Autodesk Inventor part; units mm, degrees
ref_plane "YZ Plane" through (0, 0, 0) normal (1, 0, 0) x (0, 1, 0)
ref_plane "XZ Plane" through (0, 0, 0) normal (0, 1, 0) x (-1, 0, 0)
ref_plane "XY Plane" through (0, 0, 0) normal (0, 0, 1) x (1, 0, 0)
sketch "スケッチ1" plane through (0, 0, 0) normal (0, 1, 0) x (-1, 0, 0)
  line L0 (0, 0) -> (-230, 0)
  line L1 (-230, 0) -> (-230, -35)
  line L2 (-230, -35) -> (0, -35)
  line L3 (0, -35) -> (0, 0)
  arc A0 (0, -35) -> (0, 0) centre (0, -17.5) ccw
  dimension "d0" = 230
  dimension "d1" = 35
  dimension "d2" = 17.5
extrude "押し出し1" add sketch "スケッチ1" along normal blind 3
sketch "スケッチ2" plane through (0, 3, 0) normal (0, 1, 0) x (1, 0, 0)
  line L0 (0, 17.5) -> (238.6526, 17.5)
  line L1 (0, 0) -> (230, 0)
  arc A0 (0, 35) -> (0, 0) centre (0, 17.5) ccw
  point P0 (90, 17.5)
  point P1 (100, 17.5)
  point P2 (110, 17.5)
  point P3 (120, 17.5)
  point P4 (130, 17.5)
  point P5 (140, 17.5)
  point P6 (150, 17.5)
  point P7 (160, 17.5)
  point P8 (170, 17.5)
  point P9 (180, 17.5)
  point P10 (190, 17.5)
  point P11 (200, 17.5)
  point P12 (210, 17.5)
  point P13 (-17.5, 17.5)
  point P14 (220, 17.5)
  point P15 (80, 17.5)
  dimension "d5" = 17.5
  dimension "d13" = 10
  dimension "d14" = 10
  dimension "d15" = 10
  dimension "d16" = 10
  dimension "d17" = 10
  dimension "d18" = 10
  dimension "d19" = 10
  dimension "d20" = 10
  dimension "d21" = 10
  dimension "d22" = 10
  dimension "d23" = 10
  dimension "d24" = 10
  dimension "d35" = 17.5
  dimension "d67" = 10
  dimension "d78" = 10
  dimension "d96" = 80
hole "穴1" at (90, 3, -17.5) at (100, 3, -17.5) at (110, 3, -17.5) at (120, 3, -17.5) at (130, 3, -17.5) at (140, 3, -17.5) at (150, 3, -17.5) at (160, 3, -17.5) at (170, 3, -17.5) at (180, 3, -17.5) at (190, 3, -17.5) at (200, 3, -17.5) at (210, 3, -17.5) at (220, 3, -17.5) at (80, 3, -17.5) direction (0, -1, 0) diameter 3.2 end through all
sketch "スケッチ3" plane through (0, 3, 0) normal (0, 1, 0) x (1, 0, 0)
  line L0 (230, 35) -> (0, 35)
  point P0 (0, 0)
  point P1 (0, 17.5)
  dimension "d36" = 17.5
hole "穴2" at (0, 3, -17.5) direction (0, -1, 0) diameter 16 end through all
sketch "スケッチ4" plane through (0, 3, 0) normal (0, 1, 0) x (1, 0, 0)
  circle A0 centre (0, 17.5) radius 6
  circle A1 centre (0, 17.5) radius 8
  line L0 (-0.1439, 17.5) -> (-6.5454, 17.5)
  line L1 (-6.5454, 17.5) -> (7.5104, 17.5)
  point P0 (0, 0)
  point P1 (0, 11.5)
  point P2 (6, 17.5)
  point P3 (0, 23.5)
  point P4 (-6, 17.5)
  dimension "d44" = 12
  dimension "d45" = 0
hole "穴3" [suppressed]
sketch "スケッチ5" plane through (0, 3, 0) normal (0, 1, 0) x (1, 0, 0)
  circle A0 centre (0, 17.5) radius 8
  point P0 (0, 0)
  point P1 (15.8, 7)
  point P2 (15.8, 28)
  point P3 (24.9999, 17.5)
  dimension "d53" = 10.5
  dimension "d55" = 15.8
  dimension "d56" = 15.8
  dimension "d83" = 10.5
hole "穴4" at (15.8, 3, -28) at (15.8, 3, -7) direction (0, -1, 0) diameter 3.2 end through all
sketch "スケッチ6" plane through (0, 3, 0) normal (0, 1, 0) x (1, 0, 0)
  circle A0 centre (0, 17.5) radius 8 construction
  line L0 (0, 17.5) -> (230, 17.5) construction
  line L1 (230, 0) -> (230, 35) construction
  point P0 (0, 0)
  point P1 (67, 17.5)
  point P2 (47, 17.5)
  dimension "d69" = 47
  dimension "d70" = 20
hole "穴5" at (67, 3, -17.5) at (47, 3, -17.5) direction (0, -1, 0) diameter 6.4 end through all
sketch "スケッチ7" plane through (0, 3, 0) normal (0, 1, 0) x (1, 0, 0)
  circle A0 centre (0, 17.5) radius 8 construction
  circle A1 centre (0, 17.5) radius 12.5 construction
  point P0 (0, 0)
  point P1 (0, 5)
  point P2 (12.5, 17.5)
  point P3 (0, 30)
  point P4 (-12.5, 17.5)
  dimension "d84" = 25
  dimension "d87" = 360
hole "穴6" [suppressed]
properties part number "shoulder2_lower_left_plate" material "アルミニウム 5052"
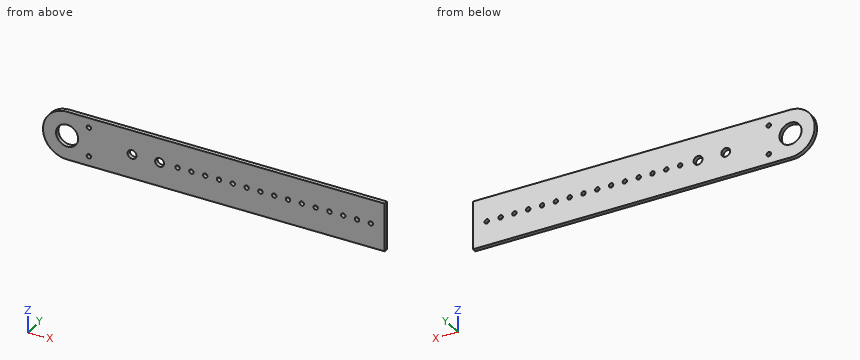
CAD build for the part. Positions are in the model's coordinates, mm. Coordinates: 2 decimals unless noted, no trailing zeros. Write each loop counter-clockwise with the first axis right and the second up, starting at its lowest first coordinate (ties: lowest second). Pieces come first, ordered by that corner, then holes. Notation, with made-up numbers: (85.25, 68) - (135.25, 68) arc R12 cw to (135.25, 80) - close; hole circle Ø1 at (62.5, 27). An arc over 180 degrees is marked (long way). Use a Markdown table: item, result. Add a question column.
Item 1: Band-saw the part on B-B, the plane y = 1.75. Give the number of separate pieces and of enclosed holes in the cut face, and give its area (3 significant figures).
Item 2: Flat gauge pin, fed straight in: pin 1 (1.9 mm diameter, centred on x = 90, z = -17.5, fed in from +Y). Where does the tip first touch, or does it go through?
Item 3: Band-saw the part on A-A, the plane x = 47. Give the cut face in (y, z).
Item 4: Drill centre lines: L1, parallel to Z at x = 47, y = 1.1; L2, parallel to Z at x = 150, y = 0.6; L3, parallel to X at y = 1.6, z = -15.5. Where is each one in solid material? Low to high. Write a range as from..to.
Item 5: Band-saw the part on C-C, the plane z = -3. Give the cut face in (x, y).
Numbers:
| question | item | result |
|---|---|---|
| 1 | separate pieces | 1 |
| 1 | enclosed holes | 20 |
| 1 | area | 8,130 mm2 |
| 2 | pin 1 | through |
| 3 | outline | (0, -35) - (3, -35) - (3, -20.7) - (0, -20.7) - close; (0, -14.3) - (3, -14.3) - (3, 0) - (0, 0) - close |
| 4 | L1 | -35..-20.7, -14.3..0 |
| 4 | L2 | -35..-19.1, -15.9..0 |
| 4 | L3 | -17.39..-7.75, 7.75..44.5, 49.5..64.5, 69.5..230 |
| 5 | outline | (-9.8, 0) - (230, 0) - (230, 3) - (-9.8, 3) - close |
